Job drawing, mm, ordinate dimensions from the low corner. One solid piece. A direction names the side the tool comes from. Give positions to 0.01 mm unless a question says otherwise; leave off trailing zeros. Order: outer loops, then holes, each group sorted by start corner. A loop starts at its lowest first (then second) coordinate and runs counter-clockwise, first axis right, second up.
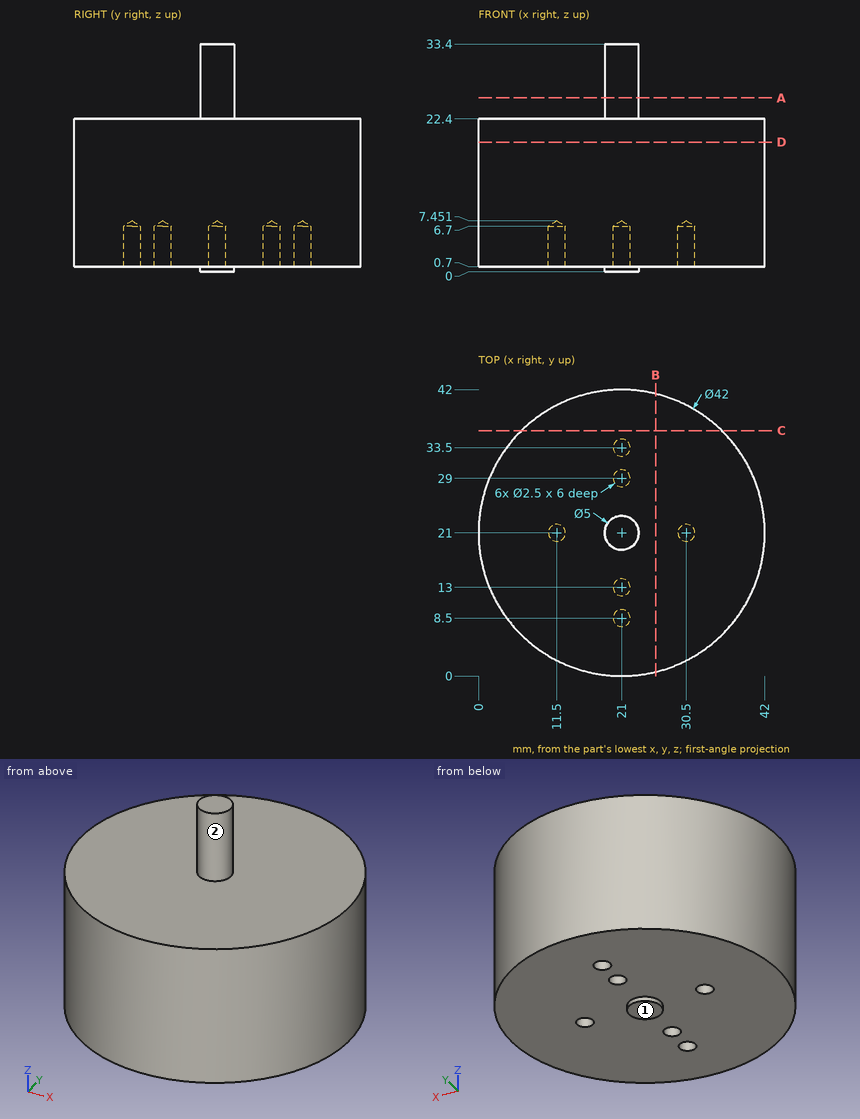
Item 1: Drill centre lines: probe 1 along Z at (x, y) = (30, 5.5); probe 2 along X at (y, z) = (29, 5.1); probe 3 along Y at (x, z) = (11.5, 5.1). Where is each one in solid material? Low to high.
Item 2: Band-saw the part on D-D on z = 19. List the corners of the cut face in (x, y), plus the area to 3 significant figures.
Item 3: Band-saw the part on C-C on y = 36. List the corners of the cut face in (x, z).
Item 4: Which spindle directions (+Z, -Z, +X, -X, +Y, -Y) get a long thin tool onto all of the face, cutting with end or side? Do the marked faces 1 and 2. Say none if no direction does.
Item 5: Band-saw the part on B-B on x = 26. List the corners of the cut face in (y, z).
Item 6: Drop flat-ended pins along their axis: P1, Ø3, axis at x = 11.5, y = 21, coming from the -Z side; P2, Ø2, axis at x = 21, y = 8.5, coming from the -Z side; P3, Ø2, axis at x = 30.5, y = 21, coming from the +Z side. Give the stop position or say it passes through.
Item 7: Band-saw the part on A-A on z = 25.5. List the corners of the cut face in (x, y), plus the area to 3 significant figures.
Working result:
1. probe 1: z = 0.7 to 22.4
1. probe 2: x = 1.58 to 19.75, 22.25 to 40.42
1. probe 3: y = 2.27 to 19.75, 22.25 to 39.73
2. outline: circle Ø42 at (21, 21)
2. area: 1,390 mm2
3. outline: (6.3, 0.7) - (35.7, 0.7) - (35.7, 22.4) - (6.3, 22.4) - close
4. face 1: -Z, +X, -X, +Y, -Y
4. face 2: +Z
5. outline: (0.6, 0.7) - (41.4, 0.7) - (41.4, 22.4) - (0.6, 22.4) - close
6. P1: stops at z = 0.7
6. P2: stops at z = 6.85
6. P3: stops at z = 22.4
7. outline: circle Ø5 at (21, 21)
7. area: 19.6 mm2
